Part model, mm, in its own coordinate system. Face numbers are marked on the shaded views. Round coordinates to 2 decimals unless told otherwise and drop trailing zeros. Loops run counter-clockwise (first coordinate to the right, second up) from the corner with the lowest first, then second, coordinate; pieces in that order, holes last. Notation, with made-up numbers: M 33,82.25 L 45,82.25 A19 cw 45,107.25 Z; hole C 76.25,25 d11. An arc over 180 degrees is marked long. Answer as CSV lines item,"result". Start each with the question number.
Item 1: Mould opens along X. For the marked faces 1, 2, 3 and 4 say: pulls with the +X half, pulls with the -X half, needs draft (parallel to the pull), parting line crosses it, or undercut.
Item 2: Band-saw the part on D-D (y = 0.75). Give the cut face in (x, z), and give its area (3 significant figures).
Item 3: Band-saw the part on B-B (y = 3.75). Give the cut face in (x, z), and give its area (3 significant figures).
Item 4: Band-saw the part on C-C (z = -0.3). Give the cut face in (x, y).
Item 5: Drop a flat-ended pin along its axis: pin 1 Ø3 at (x, y) = (-13, -1) entering from +Z. Give the stop position or say it passes through.
Item 6: Band-saw the part on A-A (x = 13.5). Give the cut face in (y, z), and give its area (3 significant figures).
Item 7: Wall check: line 1 (Y direction, x = 0, z = 0.75); line 2 (Y direction, x = 13.5, z = -0.8); line 3 (X direction, y = -4, z = -0.45). Give the ranges that are in metal, low to high.
```python
from build123d import *

# Parameters (mm, degrees)
F0_W     = 34.5
F0_H     = 12.5
F0_R     = 5
F0_R_2   = 1.65
F1_DEPTH = 2
F2_DEPTH = 2


with BuildPart() as f1:
    # F0 (on Top) → F1 (new body)
    with BuildSketch(Plane.XY):
        Rectangle(F0_W, F0_H)
        Polygon((-16.9641016151, 0), (-15.2320508076, 3), (-11.7679491924, 3), (-10.0358983849, 0), (-11.7679491924, -3), (-15.2320508076, -3), align=None, mode=Mode.SUBTRACT)
        Circle(F0_R, mode=Mode.SUBTRACT)
        Polygon((10.0358983849, 0), (11.7679491924, 3), (15.2320508076, 3), (16.9641016151, 0), (15.2320508076, -3), (11.7679491924, -3), align=None, mode=Mode.SUBTRACT)
        Polygon((-11.7679491924, 3), (-15.2320508076, 3), (-16.9641016151, 0), (-15.2320508076, -3), (-11.7679491924, -3), (-10.0358983849, 0), align=None)
        with Locations((-13.5, 0)):
            Circle(F0_R_2, mode=Mode.SUBTRACT)
        Polygon((15.2320508076, 3), (11.7679491924, 3), (10.0358983849, 0), (11.7679491924, -3), (15.2320508076, -3), (16.9641016151, 0), align=None)
        with Locations((13.5, 0)):
            Circle(F0_R_2, mode=Mode.SUBTRACT)
    extrude(amount=-F1_DEPTH)

    # F0 (on Top) → F2 (join)
    with BuildSketch(Plane.XY):
        Rectangle(F0_W, F0_H)
        Polygon((-16.9641016151, 0), (-15.2320508076, 3), (-11.7679491924, 3), (-10.0358983849, 0), (-11.7679491924, -3), (-15.2320508076, -3), align=None, mode=Mode.SUBTRACT)
        Circle(F0_R, mode=Mode.SUBTRACT)
        Polygon((10.0358983849, 0), (11.7679491924, 3), (15.2320508076, 3), (16.9641016151, 0), (15.2320508076, -3), (11.7679491924, -3), align=None, mode=Mode.SUBTRACT)
    extrude(amount=F2_DEPTH)


solid = f1.part
```
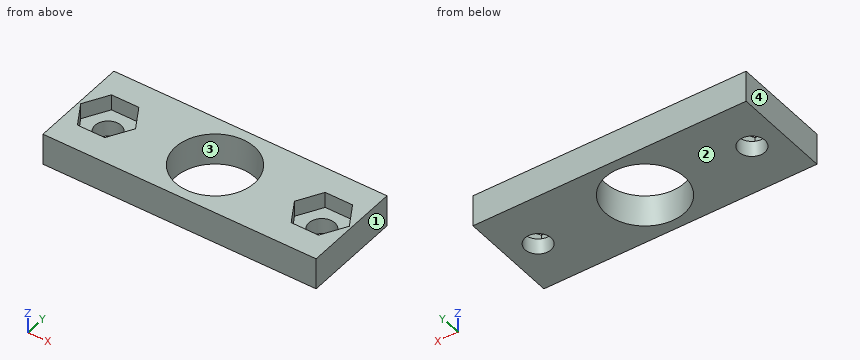
Answer block:
1,face 1,"pulls with the +X half"
1,face 2,"needs draft"
1,face 3,"undercut"
1,face 4,"pulls with the -X half"
2,outline,"M -17.25,-2 L -14.97,-2 L -14.97,0 L -16.53,0 L -16.53,2 L -17.25,2 Z; M -12.03,-2 L -4.94,-2 L -4.94,2 L -10.47,2 L -10.47,0 L -12.03,0 Z; M 4.94,-2 L 12.03,-2 L 12.03,0 L 10.47,0 L 10.47,2 L 4.94,2 Z; M 14.97,-2 L 17.25,-2 L 17.25,2 L 16.53,2 L 16.53,0 L 14.97,0 Z"
2,area,"62.4 mm^2"
3,outline,"M -17.25,-2 L -3.31,-2 L -3.31,2 L -17.25,2 Z; M 3.31,-2 L 17.25,-2 L 17.25,2 L 3.31,2 Z"
3,area,"112 mm^2"
4,outline,"M -17.25,-6.25 L 17.25,-6.25 L 17.25,6.25 L -17.25,6.25 Z; hole C -13.5,0 d3.3; hole C 0,0 d10; hole C 13.5,0 d3.3"
5,pin 1,"stops at z = 0"
6,outline,"M -6.25,-2 L -1.65,-2 L -1.65,0 L -3,0 L -3,2 L -6.25,2 Z; M 1.65,-2 L 6.25,-2 L 6.25,2 L 3,2 L 3,0 L 1.65,0 Z"
6,area,"31.4 mm^2"
7,line 1,"y = -6.25 to -5, 5 to 6.25"
7,line 2,"y = -6.25 to -1.65, 1.65 to 6.25"
7,line 3,"x = -17.25 to -3, 3 to 17.25"
